For this review, use the dimensioned drawing (mm, ordinates from the lowest corner) and the shaded views. Coordinates: 2 decimals unless noted, no trailing zeros. Loops run counter-clockwise (first coordinate to the right, second up) from the corner with the lowest first, then second, coordinate; pieces in that order, holes last. Notation, with made-up numbers: M 55.25,-7.75 L 78.25,-7.75 A30 ccw 78.25,14.25 Z; hole C 88,-30 d6. An arc over 180 degrees is marked long. One line per item, written item: value.
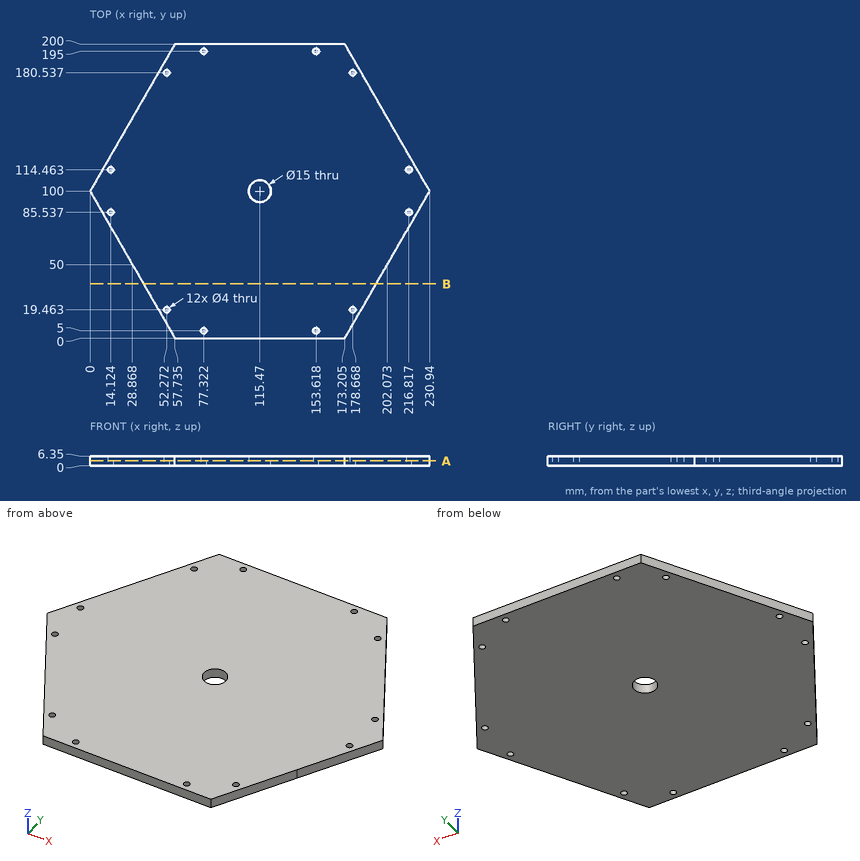
(1) Insertion check: pin 1 (2.5 mm diameter, centred on x = 14.12, y = 85.54, fed in from +Z); pin 2 (3 mm diameter, centred on x = 182, z = 1.5, fed in from +Y) (1 decimal); pin 3 (2 mm diameter, centred on y = 162, z = 4.5, fed in from -X). Each pin has a flat end and moves straight along its axis. Give the tip position at first contact, or say it passes through.
Reply:
pin 1: passes through
pin 2: stops at y = 187.4
pin 3: stops at x = 35.22
(2) To check wall thickness, follow line 1 along X through (y, z) = (86, 1.25) (1 decimal); line 2 along X through (y, z) = (5, 3.5); line 3 along X through (y, z) = (81.5, 3). State the ranges of each line that lie inside material, in increasing order. Write a range as [from, to].
Reply:
line 1: x = [8.1, 12.2], [16.1, 214.9], [218.8, 222.9]
line 2: x = [54.85, 75.32], [79.32, 151.62], [155.62, 176.09]
line 3: x = [10.68, 220.26]
(3) We need section B-B on y = 37. State the section outline as (x, z) points, then the cut area to 3 significant figures.
Reply:
outline: M 36.37,0 L 194.57,0 L 194.57,6.35 L 36.37,6.35 Z
area: 1,000 mm2
(4) We need section A-A on z = 3.25. State how many separate pieces and enclosed holes the cut face has, then the cut area to 3 significant figures.
Reply:
separate pieces: 1
enclosed holes: 13
area: 34,300 mm2
